Input: part model. Units: mm. Frame: model coordinates. A direction names the side the tool comes from. Round coordinates to 2 decimals unless told otherwise and drop trailing zeros. Loops run counter-clockwise (first coordinate to the right, second up) from the corner with the lowest first, then second, coordinate; pieces in that order, holes last.
1) First-contact query: pin 1 (1.5 mm diameter, centred on x = 69, z = 22.5, fed in from -Y); pin 2 (1.5 mm diameter, centred on y = 50, z = 23.5, fed in from +X); pin 3 (8 mm diameter, centred on y = 32.5, z = 14, fed in from +X). Flat tips, straight axial feed; report the tip coordinate or a pass-through.
2) Section A-A, the plane x = 205.5. Return loops of the section in (y, z), and give its area (3 significant figures).
3) Section C-C, the plane z = 9. Return loops of the section in (x, y), and give its area (3 significant figures).
4) Section D-D, the plane x = 147. Return loops of the section in (y, z), and give its area (3 significant figures).
5) Ray query, line 1 along X through (y, z) = (-13.5, 34.5); line 2 along X through (y, z) = (48.5, 22); line 3 along X through (y, z) = (23.5, 5). Return the intervals inside material, ascending.
6) Access query for faces 5 (the face through (165.507, 9.677, 19.72)), 6 (the face through (7.95, -26.62, 19.72)). Directions: +Z, -Z, +X, -X, +Y, -Y. A direction counts if a zero-diameter tool reaches every point of the face in a straight line with its end or side. Return the directions, or none.
7) Draft query along X for faces 1 (the face through (212.724, -31.652, 19.72)), 2 (the face through (49.678, 17.601, 19.72)), 3 (the face through (212.565, -39.391, 19.72)), 4 (the face through (104, 82.217, 20)). Return one class per face: pulls with the +X half, pulls with the -X half, needs draft (parallel to the pull), parting line crosses it, or undercut.
8) Section B-B, the plane y = 33.5. Return loops of the section in (x, z).
from build123d import *

# Parameters (mm, degrees)
SZKIC1_R                    = 8
DODANIE_WYCI_GNI_CIE1_DEPTH = 40
SZKIC2_R                    = 8
WYTNIJ_WYCI_GNI_CIE2_DEPTH  = 200


with BuildPart() as part:
    # Szkic1 → Dodanie-wyciągnięcie1 (new body)
    with BuildSketch(Plane.XY):
        with BuildLine():
            Line((3.339539238, -8.616464397), (58.496757029, 82.217181769))
            Line((58.496757029, 82.217181769), (150.074280719, 82.217181769))
            Line((150.074280719, 82.217181769), (216.294351194, -21.596573875))
            ThreePointArc((216.294351194, -21.596573875), (212.325412695, -39.547828071), (194.3741585, -35.578889572))
            Line((194.3741585, -35.578889572), (135.819853477, 56.217181769))
            Line((135.819853477, 56.217181769), (73.126827199, 56.217181769))
            Line((73.126827199, 56.217181769), (25.563122599, -22.111365012))
            ThreePointArc((25.563122599, -22.111365012), (7.703880611, -26.475706385), (3.339539238, -8.616464397))
        make_face()
        with Locations((14.451330919, -15.363914704)):
            Circle(SZKIC1_R, mode=Mode.SUBTRACT)
        with Locations((205.334254847, -28.587731723)):
            Circle(SZKIC1_R, mode=Mode.SUBTRACT)
    extrude(amount=DODANIE_WYCI_GNI_CIE1_DEPTH)

    # Szkic2 → Wytnij-wyciągnięcie2 (cut)
    with BuildSketch(Plane.XY.offset(40)):
        with Locations((66.446533252, 68.583395935)):
            Circle(SZKIC2_R)
    extrude(amount=-WYTNIJ_WYCI_GNI_CIE2_DEPTH, mode=Mode.SUBTRACT)


solid = part.part
Final values:
1. pin 1: stops at y = 48.19
1. pin 2: stops at x = 171.1
1. pin 3: stops at x = 184.34
2. outline: (-41.59, 0) - (-36.59, 0) - (-36.59, 40) - (-41.59, 40) - close; (-20.59, 0) - (-4.67, 0) - (-4.67, 40) - (-20.59, 40) - close
2. area: 837 mm2
3. outline: (3.34, -8.62) arc R13 ccw to (25.56, -22.11) - (73.13, 56.22) - (135.82, 56.22) - (194.37, -35.58) arc R13 ccw to (216.29, -21.6) - (150.07, 82.22) - (58.5, 82.22) - close; hole circle Ø16 at (14.45, -15.36); hole circle Ø16 at (66.45, 68.58); hole circle Ø16 at (205.33, -28.59)
3. area: 7,520 mm2
4. outline: (38.69, 0) - (82.22, 0) - (82.22, 40) - (38.69, 40) - close
4. area: 1,740 mm2
5. line 1: x = 1.59 to 6.67, 22.23 to 30.79, 180.29 to 211.13
5. line 2: x = 38.02 to 68.44, 140.74 to 171.58
5. line 3: x = 22.84 to 53.26, 156.69 to 187.53
6. face 5: +Z, -Z, -Y
6. face 6: +Z, -Z
7. face 1: undercut
7. face 2: undercut
7. face 3: parting line crosses it
7. face 4: needs draft
8. outline: (28.91, 0) - (59.33, 0) - (59.33, 40) - (28.91, 40) - close; (150.31, 0) - (181.15, 0) - (181.15, 40) - (150.31, 40) - close
